The drawing under review shows one solid part. Ordinate dimensions are in mm from its lowest x, y, z. A direction names the side the tool comes from. Coordinates: 2 decimals unless noted, no trailing zeros. Write each loop counter-clockwise with the first axis right and the second up, starting at its lowest first coordinate (ties: lowest second). Pieces come first, ordered by that corner, then holes. Notation, with made-up numbers: (3.25, -31) - (8.25, -31) arc R13 cw to (8.25, -6) - close; hole circle Ø4 at (14.25, 52). An arc over 180 degrees is marked (long way). Use a Markdown table: item, result.
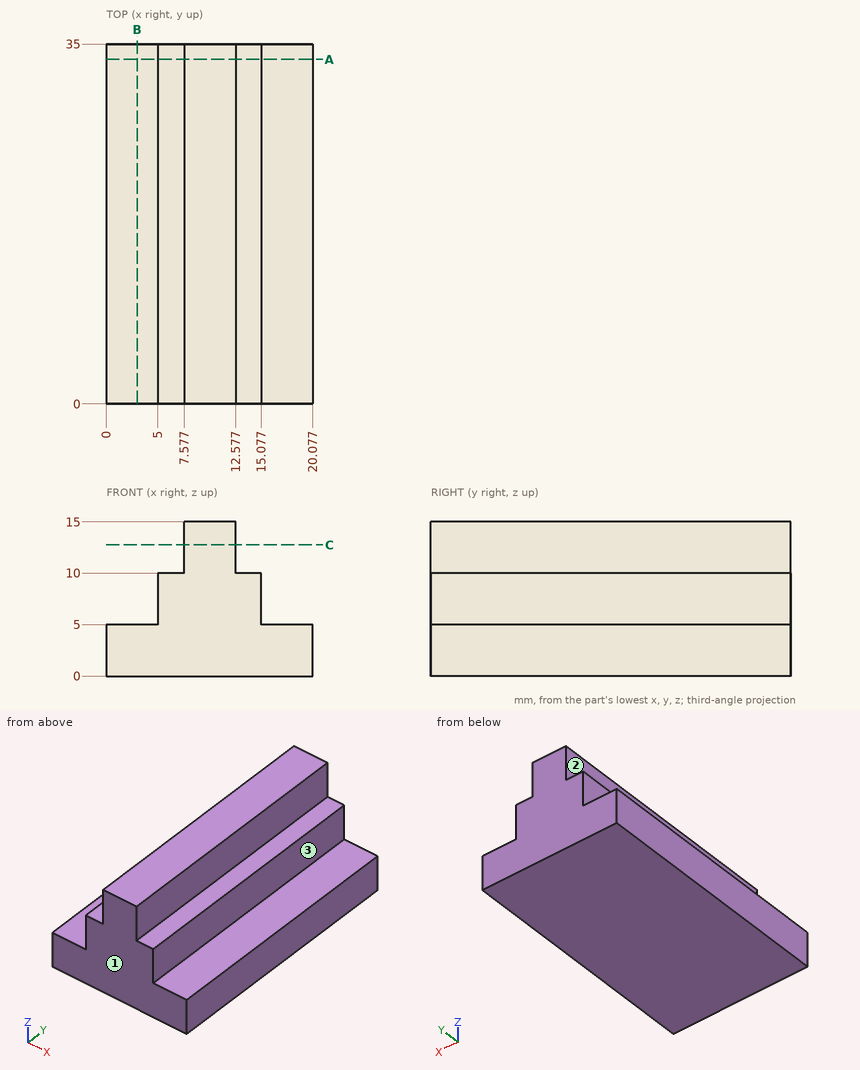
(1) Machinability: for the marked faces 1, 2 and 3, which of the approach directions +Z, -Z, +X, -X, +Y, -Y give a long, thin tool a straight path to every point of the face, cutting with its end or side? Answer none if there is none.
Determined:
| item | result |
|---|---|
| face 1 | +Z, -Z, +X, -X, -Y |
| face 2 | +Z, -X, +Y, -Y |
| face 3 | +Z, +X, +Y, -Y |
(2) Take a section at A-A on y = 33.5. Write out the cut boundary in (x, z).
Determined:
| item | result |
|---|---|
| outline | (0, 0) - (20.08, 0) - (20.08, 5) - (15.08, 5) - (15.08, 10) - (12.58, 10) - (12.58, 15) - (7.58, 15) - (7.58, 10) - (5, 10) - (5, 5) - (0, 5) - close |
(3) For L1, parallel to Z at x = 4, y = 24; L2, parallel to Z at x = 5.5, y = 19.5; L3, parallel to X at y = 33, z = 11.5, list the stretches that pass through material, from the lowest coordinate up. Write a range as from..to.
Determined:
| item | result |
|---|---|
| L1 | 0..5 |
| L2 | 0..10 |
| L3 | 7.58..12.58 |
(4) Take a section at B-B on x = 3. Write out the cut boundary in (y, z), and give its area (3 significant figures).
Determined:
| item | result |
|---|---|
| outline | (0, 0) - (35, 0) - (35, 5) - (0, 5) - close |
| area | 175 mm2 |
(5) For pin 1 (5.5 mm diameter, centred on y = 10, z = 13, fed in from +X); pin 2 (2.5 mm diameter, centred on x = 18, y = 23.5, fed in from +Z); pin 3 (1 mm diameter, centred on x = 13.5, z = 13, fed in from -Y); pin 4 (2 mm diameter, centred on x = 6, y = 15, fed in from +Z), all flat-tipped, find the tip position at first contact; note any pin that passes through.
Determined:
| item | result |
|---|---|
| pin 1 | x = 12.58 |
| pin 2 | z = 5 |
| pin 3 | through |
| pin 4 | z = 10 |
(6) Take a section at C-C on z = 12.75. Write out the cut boundary in (x, y).
Determined:
| item | result |
|---|---|
| outline | (7.58, 0) - (12.58, 0) - (12.58, 35) - (7.58, 35) - close |
